Solid Edge part; units mm, degrees
sketch "Sketch1" plane through (0, 0, 0) normal (0, -1, 0) x (1, 0, 0)
  line L0 (31.4924, 49.0939) -> (121.4924, 49.0939)
  line L1 (121.4924, 49.0939) -> (121.4924, 9.0939)
  line L2 (121.4924, 9.0939) -> (31.4924, 9.0939)
  line L3 (31.4924, 9.0939) -> (31.4924, 49.0939)
  dimension "D1" = 31.4924
  dimension "D2" = 121.4924
extrude "Protrusion1" add sketch "Sketch1" against normal blind 40
sketch "Sketch2" plane through (64.4924, 0, 22.0939) normal (0, -1, 0) x (1, 0, 0)
  line L0 (-18.0616, 9.8803) -> (-8, 10.7605)
  line L1 (-8, 10.7605) -> (-8, 18.0605)
  line L2 (-8, 18.0605) -> (34, 18.0605)
  line L3 (34, -4) -> (34, 18.0605)
  line L4 (-8, -4) -> (34, -4)
  line L5 (-8, -4) -> (-8, 3.3)
  line L6 (-8, 3.3) -> (-18.0616, 4.1803)
  line L7 (-18.0616, 4.1803) -> (-18.0616, 9.8803)
extrude "ExtrudedCutout_4" cut sketch "Sketch2" against normal blind 37
sketch "Sketch3" plane through (31.4924, 20, 22.0939) normal (-1, 0, 0) x (0, -1, 0)
  line L0 (-17, 2) -> (-17, 12)
  line L1 (-17, 12) -> (-10, 12)
  line L2 (-10, 12) -> (-10, 2)
  line L3 (-10, 2) -> (-17, 2)
  dimension "D1" = 17
  dimension "D2" = 17
  dimension "D3" = 10
extrude "Cutout1" cut sketch "Sketch3" against normal up to next
sketch "Sketch4" plane through (64.4924, 0, 22.0939) normal (0, -1, 0) x (1, 0, 0)
  line L0 (-8, 17.0605) -> (-18, 17.0605)
  line L1 (-18, 17.0605) -> (-18, -2.9395)
  line L2 (-18, -2.9395) -> (-8, -2.9395)
  line L3 (-8, -2.9395) -> (-8, 17.0605)
  line L4 (34, 17.0605) -> (44, 17.0605)
  line L5 (44, 17.0605) -> (44, -2.9395)
  line L6 (44, -2.9395) -> (34, -2.9395)
  line L7 (34, -2.9395) -> (34, 17.0605)
  dimension "D1" = 44
  dimension "D2" = 8
  dimension "D3" = 18
  dimension "D4" = 34
extrude "ExtrudedCutout_6" cut sketch "Sketch4" against normal blind 10
sketch "Sketch5" plane through (91.2324, 10, 21.645) normal (0, -1, 0) x (1, 0, 0)
  circle A0 centre (11.76, 12.5095) radius 1.65
  circle A1 centre (-39.24, 12.5095) radius 1.65
  circle A2 centre (-39.24, 2.5095) radius 1.65
  circle A3 centre (11.76, 2.5095) radius 1.65
  dimension "D1" = 39.24
  dimension "D2" = 11.76
  dimension "D3" = 39.24
extrude "Cutout2" cut sketch "Sketch5" against normal through all
sketch "Sketch6" plane through (68.9924, 0, 22.0939) normal (0, -1, 0) x (1, 0, 0)
  line L0 (-37.5, 27) -> (-37.5, -13)
  line L1 (-37.5, -13) -> (52.5, -13)
  line L2 (52.5, -13) -> (52.5, 27)
  line L3 (52.5, 27) -> (-37.5, 27)
  line L4 (-22.5616, 13.0605) -> (-22.5616, 18.0605)
  line L5 (-22.5616, 18.0605) -> (39.5, 18.0605)
  line L6 (39.5, 18.0605) -> (39.5, -4)
  line L7 (39.5, -4) -> (-22.5616, -4)
  line L8 (-22.5616, 13.0605) -> (-22.5616, -4)
  dimension "D1" = 39.5
extrude "ExtrudedProtrusion_4" add sketch "Sketch6" along normal blind 28.07
sketch "Sketch7" plane through (68.9924, -28.07, 22.0939) normal (0, -1, 0) x (1, 0, 0)
  circle A0 centre (-4.46, 7) radius 23.5
extrude "ExtrudedCutout_9" cut sketch "Sketch7" against normal blind 33.07
sketch "Sketch8" plane through (41.8429, -28.07, 29.0939) normal (0, -1, 0) x (0, 0, 1)
  line L0 (0, 10.3505) -> (5, 10.3505)
  line L1 (5, 10.3505) -> (5, -79.6495)
  line L2 (5, -79.6495) -> (0, -79.6495)
  line L3 (0, -79.6495) -> (-5, -79.6495)
  line L4 (-5, -79.6495) -> (-5, 10.3505)
  line L5 (-5, 10.3505) -> (0, 10.3505)
  dimension "D1" = 5
extrude "Cutout3" cut sketch "Sketch8" against normal blind 15
sketch "Sketch9" plane through (41.8429, -28.07, 41.5939) normal (0, -1, 0) x (0, 0, 1)
  circle A0 centre (2.5, 5.3505) radius 2.25
  circle A1 centre (-27.5, -74.6495) radius 2.25
  dimension "D1" = 2.5
extrude "ExtrudedCutout_13" cut sketch "Sketch9" against normal blind 5
sketch "Sketch10" plane through (76.4924, 5.965, 49.0939) normal (0, 0, 1) x (-1, 0, 0)
  line L0 (-0.379, 0.965) -> (24.299, 0.965)
  line L1 (24.299, 0.965) -> (45, 0.965)
  line L2 (45, 0.965) -> (55, 0.965)
  line L3 (55, 0.965) -> (55, -9.035)
  line L4 (55, -9.035) -> (45, -9.035)
  line L5 (45, -9.035) -> (-45, -9.035)
  line L6 (-45, -9.035) -> (-55, -9.035)
  line L7 (-55, -9.035) -> (-55, 0.965)
  line L8 (-55, 0.965) -> (-45, 0.965)
  line L9 (-45, 0.965) -> (-0.379, 0.965)
  dimension "D1" = 55
  dimension "D2" = 45
  dimension "D3" = 45
  dimension "D4" = 55
extrude "ExtrudedProtrusion_9" add sketch "Sketch10" against normal blind 8
sketch "Sketch11" plane through (26.4924, 10, 41.0939) normal (0, 0, -1) x (-1, 0, 0)
  circle A0 centre (0, 0) radius 2
  circle A1 centre (-100, 0) radius 2
extrude "Cutout4" cut sketch "Sketch11" against normal through all
chamfer "Chamfer_1" distance 10 angle 45 1 edges at (31.4924, 15, 45.0939)
chamfer "Chamfer_2" distance 10 angle 45 1 edges at (31.4924, 5, 45.0939)
chamfer "Chamfer_3" distance 10 angle 45 1 edges at (121.4924, 15, 45.0939)
chamfer "Chamfer_4" distance 10 angle 45 1 edges at (121.4924, 5, 45.0939)
sketch "Sketch12" plane through (76.4924, 5.965, 49.0939) normal (0, 0, 1) x (1, 0, 0)
  line L0 (-55, 9.035) -> (55, 9.035)
  line L1 (55, 9.035) -> (45, 34.035)
  line L2 (45, 34.035) -> (-45, 34.035)
  line L3 (-45, 34.035) -> (-55, 9.035)
extrude "Cutout5" cut sketch "Sketch12" against normal through all
sketch "Sketch13" plane through (99.1819, -28.07, 41.5939) normal (0, -1, 0) x (1, 0, 0)
  line L0 (-58.1495, -12.5) -> (-58.1495, 7.5)
  line L1 (-58.1495, 7.5) -> (0, 7.5)
  line L2 (0, 7.5) -> (9.3829, 7.5)
  line L3 (9.3829, 7.5) -> (9.3829, -32.5)
  line L4 (-58.1495, -32.5) -> (9.3829, -32.5)
  line L5 (-58.1495, -12.5) -> (-58.1495, -32.5)
extrude "Cutout6" cut sketch "Sketch13" against normal up to vertex (33.07 mm away)
sketch "Sketch14" plane through (36.2624, -28.07, 41.5939) normal (0, -1, 0) x (0, 0, -1)
  line L0 (2.5, -4.77) -> (2.5, 4.77)
  line L1 (2.5, 4.77) -> (7.5, 4.77)
  line L2 (7.5, 4.77) -> (7.5, -4.77)
  line L3 (7.5, -4.77) -> (2.5, -4.77)
extrude "Cutout7" cut sketch "Sketch14" against normal up to vertex (15 mm away)
sketch "Sketch15" plane through (36.2624, -28.07, 41.5939) normal (0, -1, 0) x (0, 0, -1)
  line L0 (22.5, 4.77) -> (22.5, -4.77)
  line L1 (22.5, -4.77) -> (17.5, -4.77)
  line L2 (17.5, -4.77) -> (17.5, 4.77)
  line L3 (17.5, 4.77) -> (22.5, 4.77)
extrude "Cutout8" cut sketch "Sketch15" against normal up to vertex (15 mm away)
sketch "Sketch16" plane through (36.2624, -28.07, 41.5939) normal (0, -1, 0) x (0, 0, -1)
  line L0 (2.5, 85.23) -> (7.5, 85.23)
  line L1 (7.5, 85.23) -> (7.5, 72.3024)
  line L2 (2.5, 72.3024) -> (7.5, 72.3024)
  line L3 (2.5, 85.23) -> (2.5, 72.3024)
extrude "Cutout9" cut sketch "Sketch16" against normal up to vertex (15 mm away)
sketch "Sketch17" plane through (36.2624, -28.07, 41.5939) normal (0, -1, 0) x (0, 0, -1)
  line L0 (22.5, 85.23) -> (22.5, 72.3024)
  line L1 (22.5, 72.3024) -> (17.5, 72.3024)
  line L2 (17.5, 72.3024) -> (17.5, 85.23)
  line L3 (17.5, 85.23) -> (22.5, 85.23)
extrude "Cutout10" cut sketch "Sketch17" against normal up to vertex (15 mm away)
Here's how the part is built. I have some questions about the finished solid (model axes, mm). A direction names the side the tool comes from. Coordinates: 2 decimals unless noted, no trailing zeros. Order: outer loops, then holes, each group sorted by start corner. A loop starts at its lowest first (then second) coordinate and runs counter-clockwise, first axis right, second up. Notation, with made-up numbers: (61.25, 64.25) - (76.25, 64.25) arc R30 cw to (76.25, 87.25) - close; hole circle Ø7 at (42, -30). An arc over 180 degrees is marked (long way). Use CSV: the item, a comma, the result in double quotes. Start each with the question number.
1. Suppose I cut it at C-C on z = 44. Give the number of separate pieces and of enclosed holes in the cut face, then the cut area to 3 significant figures.
2. Suppose I cut it at D-D on y = -2.5. List the corners of the cut face in (x, z) for me, then the cut area to 3 significant figures.
3. Suppose I cut it at B-B on x = 66.5. List the corners of the cut face in (y, z) for me.
4. Suppose I cut it at A-A on y = -19.5. List the corners of the cut face in (x, z) for me.
5. For faces 1 (the face through (108.492, 8, 29)), 2 (the face through (115, -21, 39.094)), 3 (the face through (41.032, -8, 29)), which set-ups out of +Z, -Z, +X, -X, +Y, -Y let a thin tool reach every point of the face, with its end or its side?
6. Please list where these lines run through material, in increasing order: line 1 (X direction, y = 2.5, z = 29.5); line 2 (Z direction, x = 67.5, y = 6); line 3 (Z direction, x = 32.5, y = -14). Write a range as from..to.
7. I'm going to push flat-ended pins straight in: pin 1 (4 mm diameter, centred on x = 55, z = 36.5, fed in from -Y); pin 2 (2 mm diameter, centred on x = 37.5, z = 43.5, fed in from -Y); pin 3 (1.5 mm diameter, centred on y = -15, z = 43.5, fed in from -X). Where does each tip first touch, or does it pass through?
8. If we mould it in two halves opening along X, with no side actions, what happens to faces 4 (the face through (51, 7, 19.154)), 5 (the face through (115, -28.07, 44))? For each: +X half, -X half, draft (parallel to the pull), parting line (faces both ways), or undercut.
Output:
1,separate pieces,"1"
1,enclosed holes,"2"
1,area,"1,900 mm2"
2,outline,"(28.99, 41.09) - (31.49, 41.09) - (31.49, 9.09) - (41.03, 9.09) - (41.03, 49.09) - (28.99, 49.09) - close; (108.56, 9.09) - (121.49, 9.09) - (121.49, 41.09) - (123.99, 41.09) - (123.99, 49.09) - (108.56, 49.09) - close"
2,area,"939 mm2"
3,outline,"(5, 9.09) - (15, 9.09) - (15, 18.09) - (5, 18.09) - close; (5, 40.15) - (15, 40.15) - (15, 49.09) - (5, 49.09) - close"
4,outline,"(31.49, 9.09) - (41.03, 9.09) - (41.03, 19.09) - (31.49, 19.09) - close; (31.49, 39.09) - (41.03, 39.09) - (41.03, 49.09) - (31.49, 49.09) - close; (108.56, 9.09) - (121.49, 9.09) - (121.49, 19.09) - (108.56, 19.09) - close; (108.56, 39.09) - (121.49, 39.09) - (121.49, 49.09) - (108.56, 49.09) - close"
5,face 1,"-Y"
5,face 2,"+X, -X, -Y"
5,face 3,"+Z, -Z, -Y"
6,line 1,"x = 31.49..41.03, 108.56..121.49"
6,line 2,"z = 9.09..18.09, 40.15..49.09"
6,line 3,"z = 9.09..19.09, 39.09..49.09"
7,pin 1,"stops at y = 10"
7,pin 2,"stops at y = -23.07"
7,pin 3,"stops at x = 31.49"
8,face 4,"undercut"
8,face 5,"draft"
